```python
from build123d import *

# Parameters (mm, degrees)
F0_R     = 2.6
F1_DEPTH = 6
F2_R     = 1


with BuildPart() as f1:
    # F0 (on Right) → F1 (new body)
    with BuildSketch(Plane.YZ):
        with BuildLine():
            ThreePointArc((10.5, 0), (0, -10.5), (-10.5, 0))
            ThreePointArc((-10.5, 0), (-16.5, 6), (-22.5, 0))
            Line((-22.5, 0), (-22.5, -15))
            ThreePointArc((-22.5, -15), (-21.035534, -18.535534), (-17.5, -20))
            Line((-17.5, -20), (17.5, -20))
            ThreePointArc((17.5, -20), (21.035534, -18.535534), (22.5, -15))
            Line((22.5, -15), (22.5, 0))
            ThreePointArc((22.5, 0), (16.5, 6), (10.5, 0))
        make_face()
        with Locations((-16.5, 0)):
            Circle(F0_R, mode=Mode.SUBTRACT)
        with Locations((16.5, 0)):
            Circle(F0_R, mode=Mode.SUBTRACT)
    extrude(amount=F1_DEPTH)

    # F2
    f2_edges = [f1.edges().sort_by_distance(p)[0] for p in [
        (6, -22.5, -7.5),
        (0, -22.5, -7.5),
    ]]
    fillet(f2_edges, radius=F2_R)


solid = f1.part
```
For this review, take the finished solid that the model builds, in its own axes (mm). Coordinates: 2 decimals unless noted, no trailing zeros. Order: outer loops, then holes, each group sorted by start corner. A loop starts at its lowest first (then second) coordinate and runs counter-clockwise, first axis right, second up. Notation, with made-up numbers: (-16.75, -20) - (16.25, -20) arc R21 cw to (16.25, 15) - close; hole circle Ø3 at (47, 81.25). An arc over 180 degrees is marked (long way). Answer as a JSON object with one key per item and string values. Group by question number.
1. We need section A-A on x = 1.7. State the section outline as (y, z) points, then the cut area to 3 significant figures.
2. We need section B-B on y = -16.5. State the section outline as (x, z) points, then the cut area to 3 significant figures.
3. We need section D-D on z = -1.5. Give the number of separate pieces and of enclosed holes in the cut face, then the cut area to 3 significant figures.
4. Clearance check with flat-ended pins moving along their axes: P1, Ø1.5, axis at x = 1.5, y = -15, coming from the +Z side; P2, Ø4, axis at y = -16.5, z = 0, coming from the -X side; P3, Ø1.5, axis at x = 4.5, z = -17.5, coming from the +Y side. State where each tip first meets the part, or that it passes through.
5. We need section C-C on y = 0. State the section outline as (x, z) points.
6. The part is to be moulded in two halves that separate along Z. For faces 1 (the cylindrical face through (0.301, -22.215, -7.605)), 2 (the cylindrical face through (3, 0.2, -10.5)), 3 (the cylindrical face through (2.96, -14.02, 0.78)), say which applies: pulls with the +Z half, pulls with the -Z half, needs draft (parallel to the pull), parting line crosses it, or undercut.
7. For probe 1 along Z at (x, y) = (4.4, 16.5); probe 2 along Y at (x, z) = (0.35, -1.5); probe 3 along Y at (x, z) = (0.95, -8.25), list the stretches that pass through material, from the lowest coordinate up.
Final values:
{
 "1": {"outline": "(-22.5, -15) arc R5 ccw to (-17.5, -20) - (17.5, -20) arc R5 ccw to (22.5, -15) - (22.5, 0) arc R6 ccw to (10.5, 0) arc R10.5 cw to (-10.5, 0) arc R6 ccw to (-22.5, 0) - close; hole circle Ø5.2 at (-16.5, 0); hole circle Ø5.2 at (16.5, 0)", "area": "787 mm²"},
 "2": {"outline": "(0, -19) arc R1 ccw to (1, -20) - (5, -20) arc R1 ccw to (6, -19) - (6, -2.6) - (0, -2.6) - close; (0, 2.6) - (6, 2.6) - (6, 5) arc R1 ccw to (5, 6) - (1, 6) arc R1 ccw to (0, 5) - close", "area": "124 mm²"},
 "3": {"separate pieces": "4", "enclosed holes": "0", "area": "92.6 mm²"},
 "4": {"P1": "z = 5.95", "P2": "through", "P3": "y = 22.18"},
 "5": {"outline": "(0, -19) arc R1 ccw to (1, -20) - (5, -20) arc R1 ccw to (6, -19) - (6, -11.5) arc R1 ccw to (5, -10.5) - (1, -10.5) arc R1 ccw to (0, -11.5) - close"},
 "6": {"face 1": "needs draft", "face 2": "pulls with the +Z half", "face 3": "undercut"},
 "7": {"probe 1": "-20 to -2.6, 2.6 to 6", "probe 2": "-22.26 to -18.62, -14.38 to -10.63, 10.63 to 14.38, 18.62 to 22.26", "probe 3": "-22.5 to -6.5, 6.5 to 22.5"}
}
